CAD build for the part. Positions are in the model's coordinates, mm. Face numbers are marked on the shaded views. A direction names the side the tool comes from. Round coordinates to 2 decimals unless told otherwise and drop trailing zeros. Loops run counter-clockwise (first coordinate to the right, second up) from the corner with the lowest first, then second, coordinate; pieces in that order, holes last. Notation, with made-up numbers: (59, 61) - (97, 61) arc R21 cw to (97, 75) - close; hole circle Ø8 at (-5, -14). An arc over 180 degrees is marked (long way). Use one line per item in the form item = value.
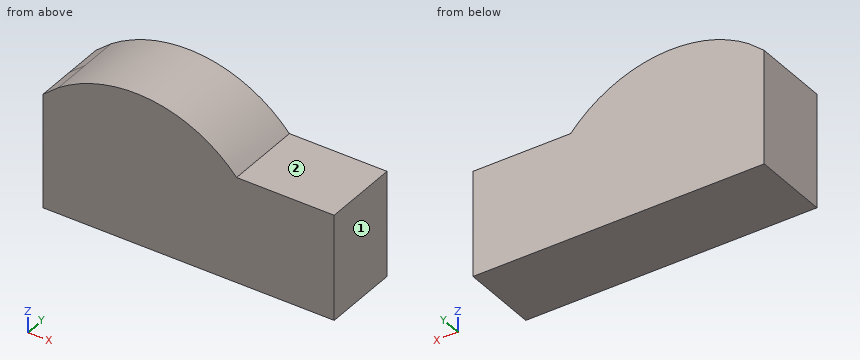
from build123d import *

# Parameters (mm, degrees)
F1_DEPTH = 12.7


with BuildPart() as f1:
    # F0 (on Front) → F1 (new body, symmetric)
    with BuildSketch(Plane.XZ):
        with BuildLine():
            Line((-63.5, 34.4180623237), (32.016806888, 34.4180623237))
            Line((32.016806888, 34.4180623237), (32.016806888, 69.0101948619))
            Line((32.016806888, 69.0101948619), (0, 69.0101948619))
            ThreePointArc((0, 69.0101948619), (-27.8940208661, 83.6123583705), (-58.4252133702, 75.9217235792))
            add(Edge.make_bspline(
                [(-63.5, 71.771000415), (-61.8079017418, 73.1557863165), (-60.1158034836, 74.540572218), (-58.4252133702, 75.9217235792)],
                knots=[0, 0, 0, 0, 0.0235260639, 0.0235260639, 0.0235260639, 0.0235260639], degree=3))
            Line((-63.5, 71.771000415), (-63.5, 34.4180623237))
        make_face()
    extrude(amount=F1_DEPTH, both=True)


solid = f1.part
1) Tool access for the marked faces 1 and 2: list every direction of +Z, -Z, +X, -X, +Y, -Y with a clear straight run to the whole face (end or side of a thin tool).
Report:
face_1 = +Z, -Z, +X, +Y, -Y
face_2 = +Z, +X, +Y, -Y
2) Flat gauge pins, fed straight in: pin 1 (8 mm diameter, centred on x = 18.5, y = 1.5, fed in from +Z); pin 2 (2 mm diameter, centred on x = -48, y = -7, fed in from +Z); pin 3 (3 mm diameter, centred on x = -44, y = 6.5, fed in from +Z). Where does each tip first touch, or does it go through?
Report:
pin_1 = 69.01
pin_2 = 81.67
pin_3 = 82.9
3) Slice it at B-B (x = -43.5). Write the cut outline in (y, z).
Report:
outline = (-12.7, 34.42) - (12.7, 34.42) - (12.7, 82.67) - (-12.7, 82.67) - close
4) Slice it at A-A (x = 3.5). Write the cut outline in (y, z).
Report:
outline = (-12.7, 34.42) - (12.7, 34.42) - (12.7, 69.01) - (-12.7, 69.01) - close
5) Drill centre lines: probe 1 along Z at (x, y) = (0, -3); probe 2 along Z at (x, y) = (-37, 10.75); probe 3 along X at (y, z) = (-7.5, 71.5). Where is each one in solid material? Low to high.
Report:
probe_1 = 34.42 to 69.01
probe_2 = 34.42 to 83.74
probe_3 = -63.5 to -2.38
